Read the model definition and answer for the solid it produces. Units are mm, in the model's axes. Face numbers are marked on the shaded views. A direction names the side the tool comes from. Give positions to 0.01 mm unless a question says otherwise; leave off trailing zeros. Loops run counter-clockwise (first coordinate to the right, second up) from the corner with the lowest first, then second, coordinate; pieces in that order, holes last. Notation, with made-up numbers: (-40, 31.25) - (5, 31.25) arc R23 cw to (5, 59.25) - close; hole circle Ø6 at (25, 78). An arc over 180 degrees is marked (long way). Use a Markdown table: item, result. Add a question column.
Item 1: Consider probe 1 along Z at (x, y) = (3, 7.5); probe 2 along Y at (x, z) = (9.5, 32); probe 3 along Y at (x, z) = (0, 14). Determine where each line is inside the solid, lowest interval first. Write a range as [from, to].
Item 2: A cutting plane is placed at B-B (z = 12). Determine the outline of the cut face in (x, y).
Item 3: A cutting plane is placed at A-A (x = 0). Determine the outline of the cut face in (y, z), plus the area to 3 significant figures.
Item 4: Each of these flat-tipped pins is pushed along its axis until it touches: P1, Ø3.5, axis at y = -1, z = 11.5, coming from the -X side; P2, Ø5, axis at x = 13, z = 17, coming from the -Y side; P3, Ø1, axis at y = -5, z = 18, coming from the +X side. Where does it stop, or does it pass through?
Item 5: A cutting plane is placed at C-C (x = 17). Determine the outline of the cut face in (y, z).
Item 6: For a pull along X with two mould halves and no side action, classify the marked faces 4, 5 and 6 as +X half, -X half, draft (parallel to the pull), parting line (faces both ways), or undercut.
Item 7: Which of the six approach directions +Z, -Z, +X, -X, +Y, -Y give full straight-line access (tool end or side, diameter ignored) to the marked faces 1, 2 and 3?
from build123d import *

# Parameters (mm, degrees)
F3_DEPTH = 1.5
F6_DEPTH = 19.5


with BuildPart() as f1:
    # F0 (on Front) → F1 (revolve)
    with BuildSketch(Plane.XZ):
        Polygon((4.2, 22.5), (4.2, 0), (13, 0), (12.9, 3.9987498046), (9, 6), (8.4, 22.5), align=None)
    revolve(axis=Axis((0, 0, 11.0757909857), (0, 0, -1)))

    # F2 (on Front) → F3 (join, symmetric)
    with BuildSketch(Plane.XZ):
        with BuildLine():
            ThreePointArc((24.8114139417, 38.3041779305), (24.1369176585, 39.5179518867), (22.8346803262, 40))
            Line((22.8346803262, 40), (7.1, 40))
            ThreePointArc((7.1, 40), (5.6857864376, 39.4142135624), (5.1, 38))
            Line((5.1, 38), (5.1, 0))
            Line((5.1, 0), (41.6566307042, 0))
            ThreePointArc((41.6566307042, 0), (46.7559189862, 2.2044542524), (48.6434507718, 7.4293545666))
            Line((48.6434507718, 7.4293545666), (48.2270230711, 14.2058177569))
            ThreePointArc((48.2270230711, 14.2058177569), (47.7443600045, 15.5294895472), (46.5087443093, 16.2064862223))
            add(Edge.make_bspline(
                [(24.8114139417, 38.3041779305), (25.8400232101, 31.6196478767), (31.7867109711, 23.9952449135), (40.4234775152, 17.0719607824), (46.5087443093, 16.2064862223)],
                knots=[0.037485554, 0.037485554, 0.037485554, 0.037485554, 0.4963538741, 0.9396396059, 0.9396396059, 0.9396396059, 0.9396396059], degree=3))
        make_face()
    extrude(amount=F3_DEPTH, both=True)

    # F5 (on offset) → F6 (join)
    with BuildSketch(Plane.XY.offset(3)):
        with BuildLine():
            Line((2.3, 3.5142566782), (2.3, -3.5142566782))
            ThreePointArc((2.3, -3.5142566782), (4.2, 0), (2.3, 3.5142566782))
        make_face()
    extrude(amount=F6_DEPTH)


solid = f1.part
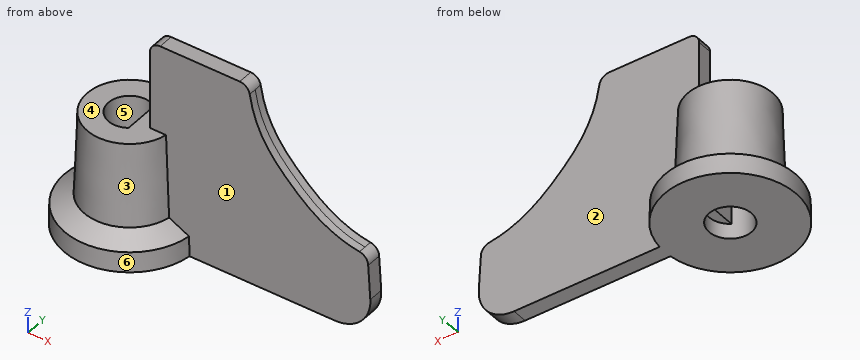
Geometry says:
| question | item | result |
|---|---|---|
| 1 | probe 1 | [0, 22.5] |
| 1 | probe 2 | [-1.5, 1.5] |
| 1 | probe 3 | [-8.71, -4.2], [4.2, 8.71] |
| 2 | outline | (8.65, -1.5) - (48.36, -1.5) - (48.36, 1.5) - (8.65, 1.5) arc R8.78 ccw (long way) to start; hole (2.3, -3.51) - (2.3, 3.51) arc R4.2 ccw (long way) to start |
| 3 | outline | (-13, 0) - (-4.2, 0) - (-4.2, 22.5) - (-8.4, 22.5) - (-9, 6) - (-12.9, 4) - close; (4.2, 0) - (13, 0) - (12.9, 4) - (9, 6) - (8.4, 22.5) - (4.2, 22.5) - close |
| 3 | area | 245 mm² |
| 4 | P1 | x = -8.85 |
| 4 | P2 | y = -1.5 |
| 4 | P3 | x = 7.29 |
| 5 | outline | (-1.5, 0) - (1.5, 0) - (1.5, 40) - (-1.5, 40) - close |
| 6 | face 4 | draft |
| 6 | face 5 | undercut |
| 6 | face 6 | parting line |
| 7 | face 1 | +Z, +X, -Y |
| 7 | face 2 | +Z, +X, +Y |
| 7 | face 3 | +Z |
